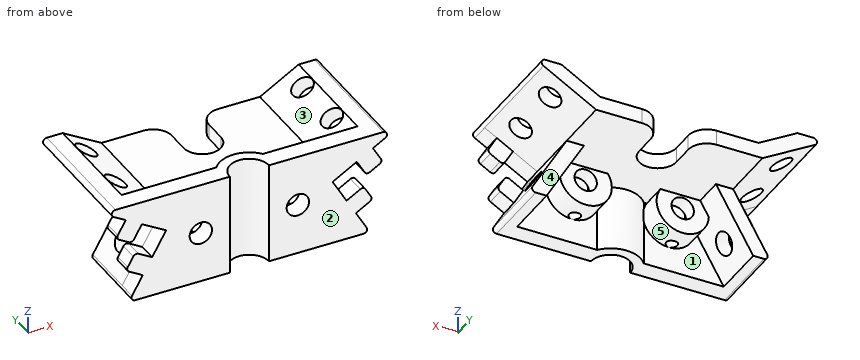
from build123d import *

# Parameters (mm, degrees)
BOSS_EXTRUDE1_DEPTH = 5
BOSS_EXTRUDE2_DEPTH = 30
BOSS_EXTRUDE3_DEPTH = 15
BOSS_EXTRUDE4_START = -27.320508
BOSS_EXTRUDE4_DEPTH = 27.320508
SKETCH6_R           = 5.25
CUT_EXTRUDE1_DEPTH  = 58.724937775
CUT_EXTRUDE2_DEPTH  = 56.139118094
SKETCH8_R           = 3
CUT_EXTRUDE3_DEPTH  = 61.901347721
SKETCH9_R           = 3
CUT_EXTRUDE4_DEPTH  = 70.587993831
SKETCH10_R          = 7
BOSS_EXTRUDE5_DEPTH = 7
SKETCH11_R          = 3
CUT_EXTRUDE5_DEPTH  = 52.343631003
CUT_EXTRUDE6_DEPTH  = 3
SKETCH14_R          = 1.5
CUT_EXTRUDE7_DEPTH  = 56.139118118


with BuildPart() as part:
    # Sketch2 → Boss-Extrude1 (new body)
    with BuildSketch(Plane(origin=(0, 0, 0), x_dir=(1, 0, 0), z_dir=(0, 1, 0))):
        with BuildLine():
            Line((-30.567949192, 27.320508076), (30.567949192, 27.320508076))
            ThreePointArc((30.567949192, 27.320508076), (31.433974596, 26.820508076), (31.433974596, 25.820508076))
            Line((31.433974596, 25.820508076), (28.55, 20.825317547))
            Line((28.55, 20.825317547), (32.230607966, 18.700317547))
            ThreePointArc((32.230607966, 18.700317547), (32.696533792, 18.093111189), (32.59663337, 17.334292144))
            Line((32.59663337, 17.334292144), (31.09663337, 14.736215932))
            ThreePointArc((31.09663337, 14.736215932), (30.489427011, 14.270290106), (29.730607966, 14.370190528))
            Line((29.730607966, 14.370190528), (26.05, 16.495190528))
            Line((26.05, 16.495190528), (22.3, 10))
            Line((22.3, 10), (28.795190528, 6.25))
            Line((28.795190528, 6.25), (30.920190528, 9.930607966))
            ThreePointArc((30.920190528, 9.930607966), (31.527396887, 10.396533792), (32.286215932, 10.29663337))
            Line((32.286215932, 10.29663337), (34.884292144, 8.79663337))
            ThreePointArc((34.884292144, 8.79663337), (35.35021797, 8.189427011), (35.250317547, 7.430607966))
            Line((35.250317547, 7.430607966), (33.125317547, 3.75))
            Line((33.125317547, 3.75), (36.388457268, 1.866025404))
            ThreePointArc((36.388457268, 1.866025404), (36.854383094, 0.741180955), (35.888457268, 0))
            Line((35.888457268, 0), (-35.888457268, 0))
            ThreePointArc((-35.888457268, 0), (-36.854383094, 0.741180955), (-36.388457268, 1.866025404))
            Line((-36.388457268, 1.866025404), (-33.125317547, 3.75))
            Line((-33.125317547, 3.75), (-35.250317547, 7.430607966))
            ThreePointArc((-35.250317547, 7.430607966), (-35.35021797, 8.189427011), (-34.884292144, 8.79663337))
            Line((-34.884292144, 8.79663337), (-32.286215932, 10.29663337))
            ThreePointArc((-32.286215932, 10.29663337), (-31.527396887, 10.396533792), (-30.920190528, 9.930607966))
            Line((-30.920190528, 9.930607966), (-28.795190528, 6.25))
            Line((-28.795190528, 6.25), (-22.3, 10))
            Line((-22.3, 10), (-26.05, 16.495190528))
            Line((-26.05, 16.495190528), (-29.730607966, 14.370190528))
            ThreePointArc((-29.730607966, 14.370190528), (-30.489427011, 14.270290106), (-31.09663337, 14.736215932))
            Line((-31.09663337, 14.736215932), (-32.59663337, 17.334292144))
            ThreePointArc((-32.59663337, 17.334292144), (-32.696533792, 18.093111189), (-32.230607966, 18.700317547))
            Line((-32.230607966, 18.700317547), (-28.55, 20.825317547))
            Line((-28.55, 20.825317547), (-31.433974596, 25.820508076))
            ThreePointArc((-31.433974596, 25.820508076), (-31.433974596, 26.820508076), (-30.567949192, 27.320508076))
        make_face()
    extrude(amount=BOSS_EXTRUDE1_DEPTH)

    # Sketch3 → Boss-Extrude2 (add)
    with BuildSketch(Plane(origin=(0, 5, 0), x_dir=(1, 0, 0), z_dir=(0, 1, 0))):
        with BuildLine():
            Line((-36.388457268, 1.866025404), (-22.3, 10))
            Line((-22.3, 10), (22.3, 10))
            Line((22.3, 10), (36.388457268, 1.866025404))
            ThreePointArc((36.388457268, 1.866025404), (36.854383094, 0.741180955), (35.888457268, 0))
            Line((35.888457268, 0), (31.620508076, 0))
            Line((31.620508076, 0), (21.22820323, 6))
            Line((21.22820323, 6), (-21.22820323, 6))
            Line((-21.22820323, 6), (-31.620508076, 0))
            Line((-31.620508076, 0), (-35.888457268, 0))
            ThreePointArc((-35.888457268, 0), (-36.854383094, 0.741180955), (-36.388457268, 1.866025404))
        make_face()
    extrude(amount=BOSS_EXTRUDE2_DEPTH)

    # Sketch4 → Boss-Extrude3 (add)
    with BuildSketch(Plane(origin=(0, 5, 0), x_dir=(1, 0, 0), z_dir=(0, 1, 0))):
        with BuildLine():
            Line((22.3, 10), (31.433974596, 25.820508076))
            ThreePointArc((31.433974596, 25.820508076), (31.433974596, 26.820508076), (30.567949192, 27.320508076))
            Line((30.567949192, 27.320508076), (27.681197846, 27.320508076))
            Line((27.681197846, 27.320508076), (17.681197846, 10))
            Line((17.681197846, 10), (22.3, 10))
        make_face()
        with BuildLine():
            Line((-27.681197846, 27.320508076), (-30.567949192, 27.320508076))
            ThreePointArc((-30.567949192, 27.320508076), (-31.433974596, 26.820508076), (-31.433974596, 25.820508076))
            Line((-31.433974596, 25.820508076), (-22.3, 10))
            Line((-22.3, 10), (-17.681197846, 10))
            Line((-17.681197846, 10), (-27.681197846, 27.320508076))
        make_face()
    extrude(amount=BOSS_EXTRUDE3_DEPTH)

    # Sketch5 → Boss-Extrude4 (add)
    with BuildSketch(Plane.XY.offset(BOSS_EXTRUDE4_START)):
        with BuildLine():
            Line((-8, 0), (8, 0))
            ThreePointArc((8, 0), (0, 8), (-8, 0))
        make_face()
    extrude(amount=BOSS_EXTRUDE4_DEPTH)

    # Sketch6 → Cut-Extrude1 (cut, through all)
    with BuildSketch(Plane.XY):
        Circle(SKETCH6_R)
    extrude(amount=-CUT_EXTRUDE1_DEPTH, mode=Mode.SUBTRACT)

    # Sketch7 → Cut-Extrude2 (cut, through all)
    with BuildSketch(Plane.XY.offset(-6)):
        with BuildLine():
            Line((-10, 35), (10, 35))
            ThreePointArc((10, 35), (6.464466094, 33.535533906), (5, 30))
            Line((5, 30), (5, 24))
            ThreePointArc((5, 24), (0, 19), (-5, 24))
            Line((-5, 24), (-5, 30))
            ThreePointArc((-5, 30), (-6.464466094, 33.535533906), (-10, 35))
        make_face()
    extrude(amount=-CUT_EXTRUDE2_DEPTH, mode=Mode.SUBTRACT)

    # Sketch8 → Cut-Extrude3 (cut, through all)
    with BuildSketch(Plane(origin=(-9.905127019, 0, -17.156183252), x_dir=(-0.8660254037844285, 0, 0.5000000000000177), z_dir=(-0.5000000000000177, 0, -0.8660254037844285))):
        with Locations((24.312366504, 28)):
            Circle(SKETCH8_R)
        with Locations((24.312366504, 13)):
            Circle(SKETCH8_R)
    cut_extrude3 = extrude(amount=-CUT_EXTRUDE3_DEPTH, mode=Mode.SUBTRACT)

    # Sketch9 → Cut-Extrude4 (cut, through all)
    with BuildSketch(Plane(origin=(-12.394872981, 0, 7.156183252), x_dir=(0.5000000000000591, 0, 0.8660254037844046), z_dir=(-0.8660254037844046, 0, 0.5000000000000591))):
        with Locations((-29.810254038, 12.5)):
            Circle(SKETCH9_R)
    cut_extrude4 = extrude(amount=-CUT_EXTRUDE4_DEPTH, mode=Mode.SUBTRACT)

    # Sketch10 → Boss-Extrude5 (add)
    with BuildSketch(Plane(origin=(0, 5, 0), x_dir=(1, 0, 0), z_dir=(0, 1, 0))):
        with Locations((-13, 13.660254038)):
            Circle(SKETCH10_R)
    boss_extrude5 = extrude(amount=BOSS_EXTRUDE5_DEPTH)

    # Sketch11 → Cut-Extrude5 (cut, through all)
    with BuildSketch(Plane(origin=(0, 12, 0), x_dir=(1, 0, 0), z_dir=(0, 1, 0))):
        with Locations(Location((-13, 13.660254038, 0), (0, 0, 270))):
            Circle(SKETCH11_R)
    cut_extrude5 = extrude(amount=-CUT_EXTRUDE5_DEPTH, mode=Mode.SUBTRACT)

    # Sketch13 → Cut-Extrude6 (cut)
    with BuildSketch(Plane(origin=(0, 5, 0), x_dir=(1, 0, 0), z_dir=(0, 1, 0))):
        Polygon((-17.25, 11.206515394), (-17.25, 6), (-8.75, 6), (-8.75, 11.206515394), (-8.75, 16.113992682), (-13, 18.567731326), (-17.25, 16.113992682), align=None)
    cut_extrude6 = extrude(amount=CUT_EXTRUDE6_DEPTH, mode=Mode.SUBTRACT)

    # Sketch14 → Cut-Extrude7 (cut, through all)
    with BuildSketch(Plane.XY.offset(-6)):
        with Locations(Location((-13, 6.5, 0), (0, 0, 270))):
            Circle(SKETCH14_R)
    cut_extrude7 = extrude(amount=-CUT_EXTRUDE7_DEPTH, mode=Mode.SUBTRACT)

    # Mirror1: Cut-Extrude3, Cut-Extrude4, Boss-Extrude5, Cut-Extrude5, Cut-Extrude6, Cut-Extrude7 across plane
    add(cut_extrude3.mirror(Plane(origin=(0, 0, 0), x_dir=(0, 0, 1), z_dir=(1, 0, 0))), mode=Mode.SUBTRACT)
    add(cut_extrude4.mirror(Plane(origin=(0, 0, 0), x_dir=(0, 0, 1), z_dir=(1, 0, 0))), mode=Mode.SUBTRACT)
    add(boss_extrude5.mirror(Plane(origin=(0, 0, 0), x_dir=(0, 0, 1), z_dir=(1, 0, 0))))
    add(cut_extrude5.mirror(Plane(origin=(0, 0, 0), x_dir=(0, 0, 1), z_dir=(1, 0, 0))), mode=Mode.SUBTRACT)
    add(cut_extrude6.mirror(Plane(origin=(0, 0, 0), x_dir=(0, 0, 1), z_dir=(1, 0, 0))), mode=Mode.SUBTRACT)
    add(cut_extrude7.mirror(Plane(origin=(0, 0, 0), x_dir=(0, 0, 1), z_dir=(1, 0, 0))), mode=Mode.SUBTRACT)


solid = part.part
Verification items for the finished model (mm, model axes). Face numbers are marked on the shaded views. A direction names the side the tool comes from. Give positions to 0.01 mm unless a question says otherwise; leave off trailing zeros. Loops run counter-clockwise (first coordinate to the right, second up) from the corner with the lowest first, then second, coordinate; pieces in that order, holes last. Notation, with made-up numbers: (53.25, 37) - (103.25, 37) arc R33 ccw to (103.25, 65) - close; hole circle Ø4 at (37, 34). An arc over 180 degrees is marked (long way). Write item = value, one per line. Start each with the question number.
Q1. Depth check by flat-ended pin: P1, Ø1.2, axis at y = 25.5, z = -8, coming from the +X side; P2, Ø1.5, axis at y = 6, z = -11, coming from the +X side; P3, Ø5, axis at x = 14.5, y = 27, coming from the -Z side. Enter the tip coordinate at first touch or a pass-through.
Q2. Cross-section at A-A, the plane x = 0. Enter the section's corners in (y, z), and give its area (3 significant figures).
Q3. Cross-section at B-B, the plane z = -19.75. State how many separate pieces and enclosed holes the cut face has, and give its area (3 significant figures).
Q4. Tool access check on the marked faces 1, 2 and 3. Record the directions out of +Z, -Z, +X, -X, +Y, -Y that give a thin tool (end or side, any length) a straight path to the whole face; none if there is none.
Q5. Thickness scan on line 1 (Z direction, x = -13, y = 2.4); line 2 (Z direction, x = -13, y = 10); line 3 (Y direction, x = -13, z = -19.5). Record the ranges inside material, lowest first.
Q6. Mould release check, pull along X, two halves, no side actions. Record for the marked faces 4 and 5: released by +X, released by -X, zero draft, split by the parting line, or undercut.
Answer key:
q1.P1 = 26.8
q1.P2 = 23.31
q1.P3 = -10
q2.outline = (5.25, -27.32) - (8, -27.32) - (8, -10) - (19, -10) - (19, -6) - (8, -6) - (8, 0) - (5.25, 0) - close
q2.area = 119 mm^2
q3.separate_pieces = 3
q3.enclosed_holes = 2
q3.area = 454 mm^2
q4.face_1 = -Z, +Y
q4.face_2 = +Z, -Z, +X, -X, -Y
q4.face_3 = +Z, +Y
q5.line_1 = -27.32 to -16.66, -10.66 to 0
q5.line_2 = -20.66 to -16.66, -10.66 to -6
q5.line_3 = 0 to 5, 8 to 12
q6.face_4 = zero draft
q6.face_5 = undercut
